The listing builds one solid part. Answer for the finished solid, in the listing's coordinates (mm). Give positions to 0.01 mm unless a question says otherwise; leave off trailing zeros. Order: outer loops, then holes, each group sorted by start corner. A loop starts at its lowest first (then second) coordinate and runs counter-clockwise, first axis right, second up. Notation, with made-up numbers: (8, 24) - (42, 24) arc R20 cw to (42, 39) - close; hole circle Ø2 at (2, 25). An arc over 180 degrees is marked (long way). Use a Markdown table: item, result. Add a question column.
1) A straight line is drawn through the part: line 1 (Y direction, x = 85.5, z = 1.4). Find the intervals that lie inside material, in ascending order.
2) Find section B-B, the plane z = 0.9. State how many separate pieces and enclosed holes the cut face has, plus the area to 3 significant figures.
3) Find section A-A, the plane x = 158. Determine the outline of the cut face in (y, z).
from build123d import *

# Parameters (mm, degrees)
MODEL_W             = 393
MODEL_H             = 170
BOSS_EXTRUDE1_DEPTH = 2
CUT_EXTRUDE1_DEPTH  = 215.105698196


with BuildPart() as part:
    # Model → Boss-Extrude1 (new body)
    with BuildSketch(Plane.XY):
        Rectangle(MODEL_W, MODEL_H)
    extrude(amount=BOSS_EXTRUDE1_DEPTH)

    # Sketch1 → Cut-Extrude1 (cut, through all)
    with BuildSketch(Plane.XY.offset(2)):
        with BuildLine():
            Line((-154.125, 43.1), (-168.4, 43.1))
            ThreePointArc((-168.4, 43.1), (-169.107106781, 43.392893219), (-169.4, 44.1))
            Line((-169.4, 44.1), (-169.4, 53.8))
            ThreePointArc((-169.4, 53.8), (-169.048528137, 54.648528137), (-168.2, 55))
            Line((-168.2, 55), (-154.325, 55))
            ThreePointArc((-154.325, 55), (-151.69102724, 53.90897276), (-150.6, 51.275))
            Line((-150.6, 51.275), (-150.6, 46.625))
            ThreePointArc((-150.6, 46.625), (-151.632448596, 44.132448596), (-154.125, 43.1))
        make_face()
        with BuildLine():
            Line((-114.125, 43.1), (-128.4, 43.1))
            ThreePointArc((-128.4, 43.1), (-129.107106781, 43.392893219), (-129.4, 44.1))
            Line((-129.4, 44.1), (-129.4, 53.8))
            ThreePointArc((-129.4, 53.8), (-129.048528137, 54.648528137), (-128.2, 55))
            Line((-128.2, 55), (-114.325, 55))
            ThreePointArc((-114.325, 55), (-111.69102724, 53.90897276), (-110.6, 51.275))
            Line((-110.6, 51.275), (-110.6, 46.625))
            ThreePointArc((-110.6, 46.625), (-111.632448596, 44.132448596), (-114.125, 43.1))
        make_face()
        with BuildLine():
            Line((-74.125, 43.1), (-88.4, 43.1))
            ThreePointArc((-88.4, 43.1), (-89.107106781, 43.392893219), (-89.4, 44.1))
            Line((-89.4, 44.1), (-89.4, 53.8))
            ThreePointArc((-89.4, 53.8), (-89.048528137, 54.648528137), (-88.2, 55))
            Line((-88.2, 55), (-74.325, 55))
            ThreePointArc((-74.325, 55), (-71.69102724, 53.90897276), (-70.6, 51.275))
            Line((-70.6, 51.275), (-70.6, 46.625))
            ThreePointArc((-70.6, 46.625), (-71.632448596, 44.132448596), (-74.125, 43.1))
        make_face()
        with BuildLine():
            Line((-34.125, 43.1), (-48.4, 43.1))
            ThreePointArc((-48.4, 43.1), (-49.107106781, 43.392893219), (-49.4, 44.1))
            Line((-49.4, 44.1), (-49.4, 53.8))
            ThreePointArc((-49.4, 53.8), (-49.048528137, 54.648528137), (-48.2, 55))
            Line((-48.2, 55), (-34.325, 55))
            ThreePointArc((-34.325, 55), (-31.69102724, 53.90897276), (-30.6, 51.275))
            Line((-30.6, 51.275), (-30.6, 46.625))
            ThreePointArc((-30.6, 46.625), (-31.632448596, 44.132448596), (-34.125, 43.1))
        make_face()
        with BuildLine():
            Line((5.875, 43.1), (-8.4, 43.1))
            ThreePointArc((-8.4, 43.1), (-9.107106781, 43.392893219), (-9.4, 44.1))
            Line((-9.4, 44.1), (-9.4, 53.8))
            ThreePointArc((-9.4, 53.8), (-9.048528137, 54.648528137), (-8.2, 55))
            Line((-8.2, 55), (5.675, 55))
            ThreePointArc((5.675, 55), (8.30897276, 53.90897276), (9.4, 51.275))
            Line((9.4, 51.275), (9.4, 46.625))
            ThreePointArc((9.4, 46.625), (8.367551404, 44.132448596), (5.875, 43.1))
        make_face()
        with BuildLine():
            Line((45.875, 43.1), (31.6, 43.1))
            ThreePointArc((31.6, 43.1), (30.892893219, 43.392893219), (30.6, 44.1))
            Line((30.6, 44.1), (30.6, 53.8))
            ThreePointArc((30.6, 53.8), (30.951471863, 54.648528137), (31.8, 55))
            Line((31.8, 55), (45.675, 55))
            ThreePointArc((45.675, 55), (48.30897276, 53.90897276), (49.4, 51.275))
            Line((49.4, 51.275), (49.4, 46.625))
            ThreePointArc((49.4, 46.625), (48.367551404, 44.132448596), (45.875, 43.1))
        make_face()
        with BuildLine():
            Line((85.875, 43.1), (71.6, 43.1))
            ThreePointArc((71.6, 43.1), (70.892893219, 43.392893219), (70.6, 44.1))
            Line((70.6, 44.1), (70.6, 53.8))
            ThreePointArc((70.6, 53.8), (70.951471863, 54.648528137), (71.8, 55))
            Line((71.8, 55), (85.675, 55))
            ThreePointArc((85.675, 55), (88.30897276, 53.90897276), (89.4, 51.275))
            Line((89.4, 51.275), (89.4, 46.625))
            ThreePointArc((89.4, 46.625), (88.367551404, 44.132448596), (85.875, 43.1))
        make_face()
        with BuildLine():
            Line((125.875, 43.1), (111.6, 43.1))
            ThreePointArc((111.6, 43.1), (110.892893219, 43.392893219), (110.6, 44.1))
            Line((110.6, 44.1), (110.6, 53.8))
            ThreePointArc((110.6, 53.8), (110.951471863, 54.648528137), (111.8, 55))
            Line((111.8, 55), (125.675, 55))
            ThreePointArc((125.675, 55), (128.30897276, 53.90897276), (129.4, 51.275))
            Line((129.4, 51.275), (129.4, 46.625))
            ThreePointArc((129.4, 46.625), (128.367551404, 44.132448596), (125.875, 43.1))
        make_face()
        with BuildLine():
            Line((165.875, 43.1), (151.6, 43.1))
            ThreePointArc((151.6, 43.1), (150.892893219, 43.392893219), (150.6, 44.1))
            Line((150.6, 44.1), (150.6, 53.8))
            ThreePointArc((150.6, 53.8), (150.951471863, 54.648528137), (151.8, 55))
            Line((151.8, 55), (165.675, 55))
            ThreePointArc((165.675, 55), (168.30897276, 53.90897276), (169.4, 51.275))
            Line((169.4, 51.275), (169.4, 46.625))
            ThreePointArc((169.4, 46.625), (168.367551404, 44.132448596), (165.875, 43.1))
        make_face()
    extrude(amount=-CUT_EXTRUDE1_DEPTH, mode=Mode.SUBTRACT)


solid = part.part
The answers:
| question | item | result |
|---|---|---|
| 1 | line 1 | -85 to 43.1, 55 to 85 |
| 2 | separate pieces | 1 |
| 2 | enclosed holes | 9 |
| 2 | area | 64,900 mm2 |
| 3 | outline | (-85, 0) - (43.1, 0) - (43.1, 2) - (-85, 2) - close; (55, 0) - (85, 0) - (85, 2) - (55, 2) - close |
